Autodesk Inventor part; units mm, degrees
ref_plane "YZ Plane" through (0, 0, 0) normal (1, 0, 0) x (0, 1, 0)
ref_plane "XZ Plane" through (0, 0, 0) normal (0, 1, 0) x (-1, 0, 0)
ref_plane "XY Plane" through (0, 0, 0) normal (0, 0, 1) x (1, 0, 0)
sketch "Sketch1" plane through (0, 0, 0) normal (0, 1, 0) x (-1, 0, 0)
  line L0 (18.5, 15.75) -> (-18.5, 15.75)
  line L1 (-18.5, 15.75) -> (-18.5, -15.75)
  line L2 (-18.5, -15.75) -> (18.5, -15.75)
  line L3 (18.5, -15.75) -> (18.5, 15.75)
  line L4 (18.5, 15.75) -> (-18.5, -15.75) construction
  line L5 (-18.5, 15.75) -> (18.5, -15.75) construction
  line L6 (0, -15.75) -> (0, -17.25)
  arc A0 (-18.5, -15.75) -> (18.5, -15.75) centre (0, 97.5833) ccw
  line L7 (-18.5, 15.75) -> (-18.5, 47.25)
  line L8 (-18.5, 47.25) -> (18.5, 47.25)
  line L9 (18.5, 47.25) -> (18.5, 15.75)
  line L10 (18.5, 15.75) -> (-18.5, 47.25) construction
  line L11 (-18.5, 15.75) -> (18.5, 47.25) construction
  line L12 (0, 47.25) -> (0, 48.75)
  arc A1 (18.5, 47.25) -> (-18.5, 47.25) centre (0, -66.0833) ccw
  point P0 (0, 0)
  point P1 (0, 31.5)
  dimension "d5" = 37
  dimension "d6" = 31.5
  dimension "d7" = 1.5
extrude "Extrusion1" add sketch "Sketch1" along normal blind 28
sketch "Sketch2" plane through (0, 0, 0) normal (0, -1, 0) x (1, 0, 0)
  arc A0 (-18.5, -15.75) -> (18.5, -15.75) centre (0, 97.5833) ccw
  line L0 (18.5, 47.25) -> (18.5, -15.75)
  line L1 (-18.5, -15.75) -> (-18.5, 47.25)
  line L2 (0, -17.25) -> (0, 58.25)
  arc A1 (18.5, 47.25) -> (-18.5, 47.25) centre (0, 37.1932) ccw
  point P0 (0, 0)
  dimension "d10" = 75.5
extrude "Extrusion2" add sketch "Sketch2" against normal blind 4
chamfer "Chamfer1" distance 2 angle 45 4 edges at (-18.5, 28, 15.75) (0, 28, 48.75) (0, 28, -17.25) (18.5, 28, 15.75)
chamfer "Chamfer2" distance 3 angle 20 1 edges at (0, 4, 58.25) measured on face at (13.1668, 2.6667, 53.6257)
sketch "Sketch3" plane through (0, 4, 0) normal (0, 1, 0) x (1, 0, 0)
  arc A0 (-17.1187, -47.4669) -> (17.1187, -47.4669) centre (0, -37.1932) ccw
  arc A1 (-17.1187, -47.4669) -> (17.1187, -47.4669) centre (0, 66.0833) ccw
  line L0 (0, -52.954) -> (0, -48.75)
  line L1 (0, -57.1581) -> (0, -52.954)
  point P0 (0, 0)
hole "Hole1" at (0, 4, 52.954) direction (0, -1, 0) diameter 4 end through all
properties part number "12v_psu"
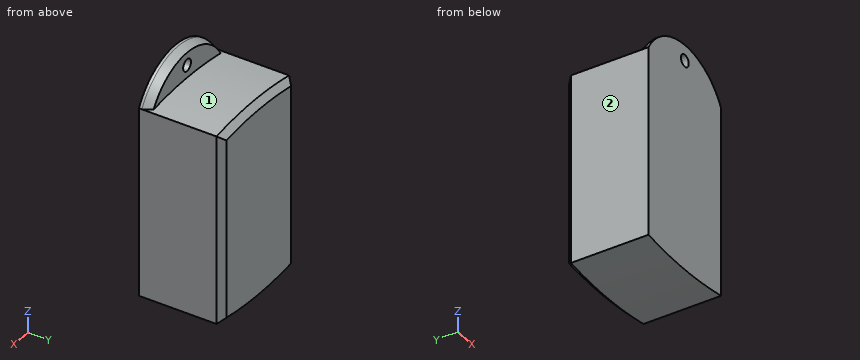
Here's how the part is built. I have some questions about the finished solid (model axes, mm). Face numbers are marked on the shaded views. A direction names the side the tool comes from. Coordinates: 2 decimals unless noted, no trailing zeros. Loops run counter-clockwise (first coordinate to the right, second up) from the corner with the lowest first, then second, coordinate; pieces in that order, holes last. Notation, with made-up numbers: (69, 14.25) - (77, 14.25) arc R25 cw to (77, 40.25) - close; hole circle Ø9 at (83, -2.75). An arc over 180 degrees is marked (long way). Answer as CSV lines item,"result".
Q1. For pin 1 (3 mm diameter, centred on x = 6, z = 53, fed in from +Y); pin 2 (3 mm diameter, centred on x = 10.5, y = 18.5, fed in from -Z); pin 3 (1 mm diameter, centred on x = 6.5, y = 16.5, fed in from -Z), each with a flat end and sliding along its axis, tell me the tip position at first contact or that it passes through.
Response:
pin 1,"y = 4"
pin 2,"z = -16.9"
pin 3,"z = -17.09"
Q2. If we section it at B-B, the plane y = 2: Write out the boundary of the cut face in (x, z).
Response:
outline,"(-18.5, -15.75) arc R114.83 ccw to (18.5, -15.75) - (18.5, 47.25) arc R114.83 ccw to (18.04, 47.32) arc R20.69 ccw to (-18.04, 47.32) arc R114.83 ccw to (-18.5, 47.25) - close; hole circle Ø4 at (0, 52.95)"
Q3. If we section it at C-C, the plane y = 17.75: Write out the boundary of the cut face in (x, z).
Response:
outline,"(-18.5, -15.75) arc R114.83 ccw to (18.5, -15.75) - (18.5, 47.25) arc R114.83 ccw to (-18.5, 47.25) - close"
Q4. If I drill on L1, parallel to Z at x = 0.5, y = 25; L2, parallel to Z at x = 0, y = 3.05; L3, parallel to Z at x = 6.5, y = 26.25, over which ranges is the centre line in solid material (lowest first)? Write a range as [from, to].
Response:
L1,"[-17.25, 48.75]"
L2,"[-17.25, 50.95], [54.95, 57.5]"
L3,"[-16.82, 48.32]"
Q5. For the marked faces 1 and 2, which set-ups out of +Z, -Z, +X, -X, +Y, -Y let a thin tool reach every point of the face, with its end or its side?
Response:
face 1,"+Z, +Y"
face 2,"+Z, -Z, -X, +Y, -Y"
Q6. If we section it at A-A, the plane x = 0: Write out the boundary of the cut face in (y, z).
Response:
outline,"(0, -17.25) - (26, -17.25) - (28, -15.25) - (28, 46.75) - (26, 48.75) - (4, 48.75) - (4, 50.95) - (0, 50.95) - close; (0, 54.95) - (4, 54.95) - (4, 57.16) - (1, 58.25) - (0, 58.25) - close"
